Build history of the part. All positions in model axes, mm. A direction names the side the tool comes from. Give positions to 0.01 mm unless a question says otherwise; leave off trailing zeros. Loops run counter-clockwise (first coordinate to the right, second up) from the corner with the lowest first, then second, coordinate; pieces in that order, holes last.
1) Flat gauge pins, fed straight in: P1, Ø6, axis at y = -338.5, z = 5, coming from the -X side; P2, Ø3, axis at x = 443, y = -33, coming from the +Z side; P3, Ø16, axis at y = -183, z = -114.5, coming from the +X side. Where does each tip first touch, or does it go through?
2) Band-saw the part on A-A on x = 450. List the corners of the cut face in (y, z), then the cut area to 3 significant figures.
3) Band-saw the part on C-C on y = -58. List the corners of the cut face in (x, z).
4) 3-axis set-ups, long thin cutter, end or side, ignore diameter. For faces 3 (the flat face through (290, -126, -109.5)), 4 (the cylindrical face through (293.428, 4.93, -88.107)), 5 (the flat face through (283.24, -39.86, -59.43)): which of +Z, -Z, +X, -X, +Y, -Y reach the whole face in a straight line?
5) Two-plate mould, pull along Y, no slides. Class faces 1 (the cylindrical face through (293.428, 4.93, -143.107)), 2 (the flat face through (35, -25, -119.5)): +Y half, -Y half, draft (parallel to the pull), parting line (faces both ways), or undercut.
6) Wall check: line 1 (X direction, y = -19, z = -22.5); line 2 (X direction, y = 3, z = -87); line 3 (Z direction, x = 615, y = 7). Give the ranges that are in metal, low to high.
7) Band-saw the part on B-B on z = 95.5. List the corners of the cut face in (x, y), then the cut area to 3 significant figures.
```python
from build123d import *

# Parameters (mm, degrees)
SKETCH_1_W             = 640
SKETCH_1_H             = 177
SKETCH_1_R             = 8.5
EXTRUDE_1_DEPTH        = 10
SKETCH_2_W             = 20
SKETCH_2_H             = 177
EXTRUDE_2_DEPTH        = 335
SKETCH_3_W             = 20
SKETCH_3_H             = 190
EXTRUDE_3_DEPTH        = 232
CUT_EXTRUDE_1_DEPTH    = 764.183464181
SKETCH_5_W             = 240
SKETCH_5_H             = 10
EXTRUDE_4_DEPTH        = 335
SKETCH_6_R             = 35
CUT_EXTRUDE_2_DEPTH    = 10
SKETCH_7_W             = 10
SKETCH_7_H             = 335
EXTRUDE_5_DEPTH        = 300
SKETCH_8_R             = 6
CUT_EXTRUDE_3_DEPTH    = 10
SKETCH_9_W             = 177
SKETCH_9_H             = 210
EXTRUDE_6_DEPTH        = 10
EXTRUDE_7_DEPTH        = 177
SKETCH_12_R            = 5
EXTRUDE_8_DEPTH        = 12
PATTERN_LINEAR_2_COUNT = 2
PATTERN_LINEAR_2_PITCH = 202
SKETCH_14_W            = 300
SKETCH_14_H            = 12
EXTRUDE_9_DEPTH        = 167
SKETCH_15_W            = 166
SKETCH_15_H            = 32
EXTRUDE_10_DEPTH       = 20
SKETCH_16_W            = 55
SKETCH_16_H            = 20
EXTRUDE_11_DEPTH       = 166
EXTRUDE_12_DEPTH       = 166
SKETCH_18_W            = 300
SKETCH_18_H            = 47
SKETCH_18_H_2          = 45
SKETCH_18_H_3          = 54
CUT_EXTRUDE_4_DEPTH    = 50
EXTRUDE_13_DEPTH       = 10
PATTERN_LINEAR_1_COUNT = 2
PATTERN_LINEAR_1_PITCH = 55
SKETCH_21_W            = 313.989613953
SKETCH_21_H            = 384
EXTRUDE_18_DEPTH       = 12


with BuildPart() as part:
    # Sketch 1 → Extrude 1 (new body)
    with BuildSketch(Plane(origin=(0, 0, 0), x_dir=(1, 0, 0), z_dir=(0, 1, 0))):
        with Locations((320, 88.5)):
            Rectangle(SKETCH_1_W, SKETCH_1_H)
        with Locations(Location((615, 142, 0), (0, 0, 270))):
            Circle(SKETCH_1_R, mode=Mode.SUBTRACT)
        with Locations(Location((615, 87, 0), (0, 0, 270))):
            Circle(SKETCH_1_R, mode=Mode.SUBTRACT)
        with Locations(Location((615, 32, 0), (0, 0, 270))):
            Circle(SKETCH_1_R, mode=Mode.SUBTRACT)
        with Locations(Location((540, 142, 0), (0, 0, 270))):
            Circle(SKETCH_1_R, mode=Mode.SUBTRACT)
        with Locations(Location((450, 142, 0), (0, 0, 270))):
            Circle(SKETCH_1_R, mode=Mode.SUBTRACT)
        with Locations(Location((360, 142, 0), (0, 0, 270))):
            Circle(SKETCH_1_R, mode=Mode.SUBTRACT)
        with Locations(Location((285, 142, 0), (0, 0, 270))):
            Circle(SKETCH_1_R, mode=Mode.SUBTRACT)
        with Locations(Location((285, 32, 0), (0, 0, 270))):
            Circle(SKETCH_1_R, mode=Mode.SUBTRACT)
        with Locations(Location((285, 87, 0), (0, 0, 270))):
            Circle(SKETCH_1_R, mode=Mode.SUBTRACT)
    extrude(amount=EXTRUDE_1_DEPTH)

    # Sketch 2 → Extrude 2 (add)
    with BuildSketch(Plane.XZ):
        with Locations((580, -88.5)):
            Rectangle(SKETCH_2_W, SKETCH_2_H)
        with Locations((320, -88.5)):
            Rectangle(SKETCH_2_W, SKETCH_2_H)
    extrude(amount=EXTRUDE_2_DEPTH)

    # Sketch 3 → Extrude 3 (add)
    with BuildSketch(Plane.XY):
        with Locations((580, -240)):
            Rectangle(SKETCH_3_W, SKETCH_3_H)
        with Locations((320, -240)):
            Rectangle(SKETCH_3_W, SKETCH_3_H)
    extrude(amount=EXTRUDE_3_DEPTH)

    # Sketch 4 → Cut-Extrude 1 (cut, through all)
    with BuildSketch(Plane.XZ.offset(335)):
        Polygon((330, 232), (320, 232), (330, 197), align=None)
        Polygon((570, 232), (580, 232), (570, 197), align=None)
    extrude(amount=-CUT_EXTRUDE_1_DEPTH, mode=Mode.SUBTRACT)

    # Sketch 5 → Extrude 4 (add)
    with BuildSketch(Plane(origin=(0, 0, 0), x_dir=(-1, 0, 0), z_dir=(0, -1, 0))):
        with Locations((-450, 172)):
            Rectangle(SKETCH_5_W, SKETCH_5_H)
    extrude(amount=EXTRUDE_4_DEPTH)

    # Sketch 6 → Cut-Extrude 2 (cut)
    with BuildSketch(Plane(origin=(0, 0, -177), x_dir=(-1, 0, 0), z_dir=(0, 0, -1))):
        with Locations((-450, -225)):
            Circle(SKETCH_6_R)
    extrude(amount=-CUT_EXTRUDE_2_DEPTH, mode=Mode.SUBTRACT)

    # Sketch 7 → Extrude 5 (add)
    with BuildSketch(Plane.ZY.offset(-310)):
        with Locations((-172, -167.5)):
            Rectangle(SKETCH_7_W, SKETCH_7_H)
    extrude(amount=EXTRUDE_5_DEPTH)

    # Sketch 8 → Cut-Extrude 3 (cut)
    with BuildSketch(Plane(origin=(0, 0, -177), x_dir=(-1, 0, 0), z_dir=(0, 0, -1))):
        with Locations((-217, -76)):
            Circle(SKETCH_8_R)
        with Locations((-103, -76)):
            Circle(SKETCH_8_R)
        with Locations((-217, -119)):
            Circle(SKETCH_8_R)
        with Locations((-103, -119)):
            Circle(SKETCH_8_R)
        Polygon((-10, -211), (-295, -335), (-10, -335), align=None)
    extrude(amount=-CUT_EXTRUDE_3_DEPTH, mode=Mode.SUBTRACT)

    # Sketch 9 → Extrude 6 (add)
    with BuildSketch(Plane.ZY.offset(-10)):
        with Locations((-88.5, -105)):
            Rectangle(SKETCH_9_W, SKETCH_9_H)
    extrude(amount=EXTRUDE_6_DEPTH)

    # Sketch 12 → Extrude 8 (add)
    with BuildSketch(Plane.XY.offset(180)):
        with BuildLine():
            Line((330, -335), (570, -335))
            Line((570, -335), (570, -145))
            Line((570, -145), (477.5, -145))
            Line((477.5, -145), (477.5, -225))
            ThreePointArc((477.5, -225), (450, -252.5), (422.5, -225))
            Line((422.5, -225), (422.5, -145))
            Line((422.5, -145), (330, -145))
            Line((330, -145), (330, -335))
        make_face()
        with Locations((405, -182)):
            Circle(SKETCH_12_R, mode=Mode.SUBTRACT)
        with Locations((495, -182)):
            Circle(SKETCH_12_R, mode=Mode.SUBTRACT)
    extrude_8 = extrude(amount=EXTRUDE_8_DEPTH)

    # Pattern Linear 2: Extrude 8 ×2
    with Locations(*[(0, 0, -i * PATTERN_LINEAR_2_PITCH) for i in range(1, PATTERN_LINEAR_2_COUNT)]):
        add(extrude_8)

    # Sketch 14 → Extrude 9 (add)
    with BuildSketch(Plane.XY.offset(-167)):
        with Locations((160, -204)):
            Rectangle(SKETCH_14_W, SKETCH_14_H)
    extrude(amount=EXTRUDE_9_DEPTH)

    # Sketch 15 → Extrude 10 (add)
    with BuildSketch(Plane(origin=(10, 0, 0), x_dir=(0, 0, -1), z_dir=(1, 0, 0))):
        with Locations((83.5, -182)):
            Rectangle(SKETCH_15_W, SKETCH_15_H)
    extrude(amount=EXTRUDE_10_DEPTH)

    # Sketch 16 → Extrude 11 (add)
    with BuildSketch(Plane.XY.offset(-0.5)):
        Polygon((310, -146), (310, -198), (290, -198), (290, -166), (255, -166), (255, -146), align=None)
        with Locations((37.5, -156)):
            Rectangle(SKETCH_16_W, SKETCH_16_H)
    extrude(amount=-EXTRUDE_11_DEPTH)

    # Sketch 17 → Extrude 12 (add)
    with BuildSketch(Plane.XY.offset(-0.5)):
        Polygon((10, -146), (60, -146), (60, -136), (30, -96), (10, -96), align=None)
        Polygon((310, -146), (260, -146), (260, -136), (290, -96), (310, -96), align=None)
    extrude(amount=-EXTRUDE_12_DEPTH)

    # Sketch 18 → Cut-Extrude 4 (cut)
    with BuildSketch(Plane(origin=(0, -96, 0), x_dir=(1, 0, 0), z_dir=(0, 1, 0))):
        with Locations((160, 143)):
            Rectangle(SKETCH_18_W, SKETCH_18_H)
        with Locations((160, 87)):
            Rectangle(SKETCH_18_W, SKETCH_18_H_2)
        with Locations((160, 27.5)):
            Rectangle(SKETCH_18_W, SKETCH_18_H_3)
    extrude(amount=-CUT_EXTRUDE_4_DEPTH, mode=Mode.SUBTRACT)

    # Sketch 20 → Extrude 13 (add)
    with BuildSketch(Plane.XY.offset(-54.5)):
        Polygon((590, 0), (640, 0), (640, -30), (610, -50), (590, -50), align=None)
        Polygon((310, 0), (276.666666667, 0), (276.666666667, -30), (290, -50), (310, -50), align=None)
        Polygon((10, 0), (10, -50), (30, -50), (60, -30), (60, 0), align=None)
    extrude_13 = extrude(amount=-EXTRUDE_13_DEPTH)

    # Pattern Linear 1: Extrude 13 ×2
    with Locations(*[(0, 0, -i * PATTERN_LINEAR_1_PITCH) for i in range(1, PATTERN_LINEAR_1_COUNT)]):
        add(extrude_13)



with BuildPart() as body_2:
    # Sketch 11 → Extrude 7 (new body)
    with BuildSketch(Plane(origin=(0, 0, -177), x_dir=(-1, 0, 0), z_dir=(0, 0, -1))):
        Polygon((-7.71078258, -210.003989614), (-295, -335), (-291.010386047, -344.16967723), (-3.71199895, -219.16967723), (-7.697623289, -210.009169677), align=None)
    extrude(amount=-EXTRUDE_7_DEPTH)


with BuildPart() as part_1:
    add(part.part)

    add(body_2.part)  # Extrude 18 merges body 2
    # Sketch 21 → Extrude 18 (add)
    with BuildSketch(Plane(origin=(0, -335, 0), x_dir=(-1, 0, 0), z_dir=(0, -1, 0))):
        with Locations((-448.005193023, -15)):
            Rectangle(SKETCH_21_W, SKETCH_21_H)
    extrude(amount=EXTRUDE_18_DEPTH)


solid = part_1.part
```
Findings below:
1. P1: stops at x = 291.01
1. P2: stops at z = -167
1. P3: stops at x = 590
2. outline: (-347, -177) - (-260, -177) - (-260, -167) - (-335, -167) - (-335, -22) - (-252.5, -22) - (-252.5, -10) - (-335, -10) - (-335, 180) - (-252.5, 180) - (-252.5, 192) - (-335, 192) - (-335, 207) - (-347, 207) - close; (-190, -177) - (10, -177) - (10, -150.5) - (0, -150.5) - (0, -167) - (-190, -167) - close; (0, -133.5) - (10, -133.5) - (10, 0) - (0, 0) - close
2. area: 10,800 mm2
3. outline: (0, -177) - (590, -177) - (590, 0) - (570, 0) - (570, -167) - (330, -167) - (330, 0) - (310, 0) - (310, -167) - (10, -167) - (10, 0) - (0, 0) - close
4. face 3: none
4. face 4: +Y
4. face 5: +Z
5. face 1: draft
5. face 2: undercut
6. line 1: x = 0 to 10, 310 to 330, 570 to 590
6. line 2: x = 0 to 276.5, 293.5 to 606.5, 623.5 to 640
6. line 3: z = -177 to -150.5, -133.5 to -95.5, -78.5 to -40.5, -23.5 to 0
7. outline: (291.01, -347) - (605, -347) - (605, -335) - (590, -335) - (590, -145) - (570, -145) - (570, -335) - (330, -335) - (330, -145) - (310, -145) - (310, -335) - (291.01, -335) - close
7. area: 11,400 mm2
